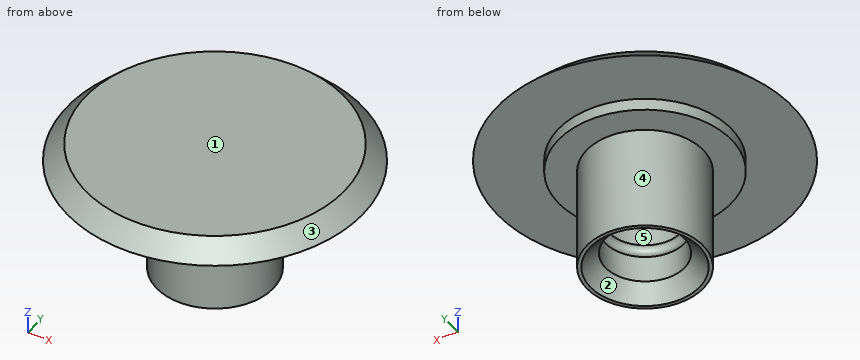
from build123d import *

# Parameters (mm, degrees)
F2_SIZE  = 1.27
F3_R     = 18.9556070846
F3_R_2   = 5.842
F4_DEPTH = 0.8
F5_SIZE  = 1.016


# Not quite as in the source:
# - a fillet or chamfer that OpenCascade refuses, or shapes differently, is made with other operations: its cross-section is extruded or revolved along the edge and cut away or added


with BuildPart() as f1:
    # F0 (on Front) → F1 (revolve)
    with BuildSketch(Plane.XZ):
        with BuildLine():
            Line((0, 0), (2.6757909362, 0))
            Line((2.6757909362, 0), (2.6757909362, -3.438))
            ThreePointArc((2.6757909362, -3.438), (2.2947909362, -3.819), (2.6757909362, -4.2))
            Line((2.6757909362, -4.2), (2.6757909362, -7))
            Line((2.6757909362, -7), (3.937, -7))
            Line((3.937, -7), (3.937, 0))
            Line((3.937, 0), (10, 0))
            Line((10, 0), (10, 2.032))
            Line((10, 2.032), (0, 2.032))
            Line((0, 2.032), (0, 0))
        make_face()
    revolve(axis=Axis((0, 0, 1.016), (0, 0, -1)))

    # F2
    f2_edges = [f1.edges().sort_by_distance(p)[0] for p in [
        (-2.675791, 0, 0),
    ]]
    chamfer(f2_edges, length=F2_SIZE)

    # F3 (on face) → F4 (cut)
    with BuildSketch(Plane(origin=(0, 0, 0), x_dir=(1, 0, 0), z_dir=(0, 0, -1))):
        with Locations((0, -0.8832210264)):
            Circle(F3_R)
        Circle(F3_R_2, mode=Mode.SUBTRACT)
    extrude(amount=-F4_DEPTH, mode=Mode.SUBTRACT)

    # F5
    f5_edges = [f1.edges().sort_by_distance(p)[0] for p in [
        (-2.675791, 0, -7),
    ]]
    chamfer(f5_edges, length=F5_SIZE)

    # F6: chamfer of 1.27 on 1 edges, made by hand

    # F6_s1 → F6_t2 (revolve, cut)
    with BuildSketch(Plane.XZ):
        Polygon((10, 0.762), (8.73, 2.032), (10, 2.032), align=None)
    revolve(axis=Axis((0, 0, 2.032), (0, 0, -1)), mode=Mode.SUBTRACT)


solid = f1.part
Source: CAD feature listing. Evaluate the final solid. Frame: model axes, mm. Face numbers are marked on the shaded views. A direction names the side the tool comes from. Coordinates: 2 decimals unless noted, no trailing zeros. Loops run counter-clockwise (first coordinate to the right, second up) from the corner with the lowest first, then second, coordinate; pieces in that order, holes last. Notation, with made-up numbers: (65.25, 49.25) -> (106.25, 49.25) arc R9 cw to (106.25, 61.25) -> close; hole circle Ø10 at (-34, -22.75). An arc over 180 degrees is marked (long way). Answer in a Markdown table with one row per item. Add a question column.
Q1. Pull-direction query (Y, two-part tool) for the marked faces 1, 2 and 3; classes: pulls with the +Y half, pulls with the -Y half, needs draft (parallel to the pull), parting line crosses it, or undercut.
Q2. Section C-C on z = -3.75. Return the cut outline in (x, y), and give its area (3 significant figures).
Q3. Contact query for flat-ended pins moving along their axis: pin 1 Ø3 at (y, z) = (-4.5, -3.5) entering from +X; pin 2 Ø2 at (x, y) = (0, -0.5) entering from -Z; pin 3 Ø6 at (x, y) = (0, 0) entering from -Z; pin 4 Ø4 at (x, y) = (3.5, -3) entering from -Z. Output: stop coordinate, or through.
Q4. Reachability of the marked faces 4 and 5 from +Z, -Z, +X, -X, +Y, -Y: full face, straight path, thin tool, end or side. Return the list, or none.
Q5. Section D-D on z = -0.5. Return the cut outline in (x, y), and give its area (3 significant figures).
Q6. Section A-A on x = 0. Return the cut outline in (y, z), and give its area (3 significant figures).
Q7. Ray query, line 1 along Y through (x, z) = (0, -5.35); line 2 along Z through (x, y) = (5.5, -4.75). Return the intervals inside material, ascending.
Computed values:
| question | item | result |
|---|---|---|
| 1 | face 1 | needs draft |
| 1 | face 2 | undercut |
| 1 | face 3 | parting line crosses it |
| 2 | outline | circle Ø7.87 at (0, 0); hole circle Ø4.6 at (0, 0) |
| 2 | area | 32.1 mm^2 |
| 3 | pin 1 | stops at x = 2.55 |
| 3 | pin 2 | stops at z = -0.09 |
| 3 | pin 3 | stops at z = -6.31 |
| 3 | pin 4 | stops at z = -7 |
| 4 | face 4 | -Z |
| 4 | face 5 | none |
| 5 | outline | circle Ø7.87 at (0, 0); hole circle Ø3.81 at (0, 0) |
| 5 | area | 37.3 mm^2 |
| 6 | outline | (-9.96, 0.8) -> (-5.84, 0.8) -> (-5.84, 0) -> (-3.94, 0) -> (-3.94, -7) -> (-3.69, -7) -> (-2.68, -5.98) -> (-2.68, -4.2) arc R0.38 ccw to (-2.68, -3.44) -> (-2.68, -1.27) -> (-1.41, 0) -> (1.41, 0) -> (2.68, -1.27) -> (2.68, -3.44) arc R0.38 ccw to (2.68, -4.2) -> (2.68, -5.98) -> (3.69, -7) -> (3.94, -7) -> (3.94, 0) -> (5.84, 0) -> (5.84, 0.8) -> (9.96, 0.8) -> (8.73, 2.03) -> (-8.73, 2.03) -> close |
| 6 | area | 51.1 mm^2 |
| 7 | line 1 | y = -3.94 to -2.68, 2.68 to 3.94 |
| 7 | line 2 | z = 0.8 to 2.03 |
